```python
from build123d import *

# Parameters (mm, degrees)
SKETCH1_W           = 90
SKETCH1_H           = 33
BOSS_EXTRUDE1_DEPTH = 64
CUT_EXTRUDE3_REACH  = 113.714
SKETCH2_W           = 26
SKETCH2_H           = 14
SKETCH3_W           = 28
SKETCH3_H           = 8.692638167
CUT_EXTRUDE4_DEPTH  = 16


with BuildPart() as part:
    # Sketch1 → Boss-Extrude1 (new body)
    with BuildSketch(Plane.XY):
        with Locations((-19.35, 0.353571429)):
            Rectangle(SKETCH1_W, SKETCH1_H)
    extrude(amount=-BOSS_EXTRUDE1_DEPTH)

    # Sketch2 → Cut-Extrude3 (cut, up to next)
    with BuildSketch(Plane(origin=(25.65, 0, 0), x_dir=(0, 0, -1), z_dir=(1, 0, 0)), mode=Mode.PRIVATE) as cut_extrude3_sk1:
        with Locations((32, -9.146428571)):
            Rectangle(SKETCH2_W, SKETCH2_H)
    cut_extrude3_tool1 = extrude(cut_extrude3_sk1.sketch, amount=-CUT_EXTRUDE3_REACH, mode=Mode.PRIVATE) & part.part
    add(cut_extrude3_tool1.solids().sort_by_distance((25.65, -9.146429, -32))[0], mode=Mode.SUBTRACT)

    # Sketch3 → Cut-Extrude4 (cut)
    with BuildSketch(Plane(origin=(0, 0, -64), x_dir=(-1, 0, 0), z_dir=(0, 0, -1))):
        with Locations((19.35, 12.507252346)):
            Rectangle(SKETCH3_W, SKETCH3_H)
    extrude(amount=-CUT_EXTRUDE4_DEPTH, mode=Mode.SUBTRACT)


solid = part.part
```
Design review of the part built by this model. Coordinates are the model's own, in mm. A direction names the side the tool comes from. Coordinates: 2 decimals unless noted, no trailing zeros. Loops run counter-clockwise (first coordinate to the right, second up) from the corner with the lowest first, then second, coordinate; pieces in that order, holes last. Notation, with made-up numbers: (-14, 84.25) -> (6, 84.25) arc R14 ccw to (6, 90.25) -> close; hole circle Ø9 at (67.25, -10). An arc over 180 degrees is marked (long way). Answer as a JSON object with one key per item and string values.
Q1. The part is to be moulded in two halves that separate along Z. For faces 4 (the flat face through (-20, -16.146, -54)), 5 (the flat face through (-20, 1, -64)), 6 (the flat face through (-19, -9, -45)), 7 (the flat face through (-19, -2.146, -32)), say which applies: +Z half, -Z half, draft (parallel to the pull), parting line (faces both ways), or undercut.
Answer block:
{"face 4": "draft", "face 5": "-Z half", "face 6": "undercut", "face 7": "undercut"}
Q2. Take a section at C-C on x = -51.5. Give the boundary of the cut face in (y, z), plus the area to 3 significant figures.
Answer block:
{"outline": "(-16.15, -64) -> (16.85, -64) -> (16.85, 0) -> (-16.15, 0) -> (-16.15, -19) -> (-2.15, -19) -> (-2.15, -45) -> (-16.15, -45) -> close", "area": "1,750 mm^2"}
Q3. Clearance check with flat-ended pins moving along their axes: pin 1 Ø5 at (x, z) = (-22.5, -59) entering from +Y; pin 2 Ø8 at (x, z) = (-24, -31) entering from -Y; pin 3 Ø4.5 at (x, y) = (-25.5, 10.5) entering from -Z. State where each tip first meets the part, or that it passes through.
Answer block:
{"pin 1": "stops at y = 8.16", "pin 2": "stops at y = -2.15", "pin 3": "stops at z = -48"}
Q4. Take a section at A-A on y = -9.5. Give the boundary of the cut face in (x, z).
Answer block:
{"outline": "(-64.35, -64) -> (25.65, -64) -> (25.65, -45) -> (-64.35, -45) -> close; (-64.35, -19) -> (25.65, -19) -> (25.65, 0) -> (-64.35, 0) -> close"}
Q5. Take a section at B-B on z = -52. Give the boundary of the cut face in (x, y), plus the area to 3 significant figures.
Answer block:
{"outline": "(-64.35, -16.15) -> (25.65, -16.15) -> (25.65, 16.85) -> (-5.35, 16.85) -> (-5.35, 8.16) -> (-33.35, 8.16) -> (-33.35, 16.85) -> (-64.35, 16.85) -> close", "area": "2,730 mm^2"}
Q6. Take a section at D-D on x = -6.5. Give the boundary of the cut face in (y, z).
Answer block:
{"outline": "(-16.15, -64) -> (8.16, -64) -> (8.16, -48) -> (16.85, -48) -> (16.85, 0) -> (-16.15, 0) -> (-16.15, -19) -> (-2.15, -19) -> (-2.15, -45) -> (-16.15, -45) -> close"}
Q7. To check wall thickness, follow L1, parallel to Z at x = -35, y = -3.5; L2, parallel to Y at x = -14, z = -22. State the ranges of each line that lie inside material, in increasing order.
Answer block:
{"L1": "z = -64 to -45, -19 to 0", "L2": "y = -2.15 to 16.85"}
Q8. Tool access review of faces 1 (the flat face through (-64.35, 0, -32)), 2 (the flat face through (-19, -9, -19)), 3 (the flat face through (-5.35, 12, -56)): name each direction out of +Z, -Z, +X, -X, +Y, -Y from which nothing blocks a thin tool from reaching the whole face with its end or side.
Answer block:
{"face 1": "+Z, -Z, -X, +Y, -Y", "face 2": "+X, -X, -Y", "face 3": "-Z, +Y"}
